```python
from build123d import *

# Parameters (mm, degrees)
SKETCH_1_W      = 180
SKETCH_1_H      = 98
SKETCH_1_R      = 6.2
SKETCH_1_R_2    = 8.2
SKETCH_1_R_3    = 1.5
SKETCH_1_R_4    = 1.75
SKETCH_1_R_5    = 3.6
SKETCH_1_R_6    = 3.8
SKETCH_1_W_2    = 12.5
SKETCH_1_H_2    = 12.5
SKETCH_1_W_3    = 46.5
SKETCH_1_H_3    = 36
EXTRUDE_1_DEPTH = 2.2
FILLET_1_R      = 1
FILLET_2_R      = 0.5


with BuildPart() as part:
    # Эскиз1 → Бобышка-Вытянуть1 (new body)
    with BuildSketch(Plane.XY):
        with Locations((49.911, 29.5)):
            Rectangle(SKETCH_1_W, SKETCH_1_H)
        with Locations((-24.089, 5.5)):
            Circle(SKETCH_1_R, mode=Mode.SUBTRACT)
        with Locations((123.911, 58.5)):
            Circle(SKETCH_1_R, mode=Mode.SUBTRACT)
        with Locations((123.911, 5.5)):
            Circle(SKETCH_1_R_2, mode=Mode.SUBTRACT)
        with Locations((-37.589, 76)):
            Circle(SKETCH_1_R_3, mode=Mode.SUBTRACT)
        with Locations((137.411, 76)):
            Circle(SKETCH_1_R_3, mode=Mode.SUBTRACT)
        with Locations((137.411, -17)):
            Circle(SKETCH_1_R_3, mode=Mode.SUBTRACT)
        with Locations((-37.589, -17)):
            Circle(SKETCH_1_R_3, mode=Mode.SUBTRACT)
        with Locations((3.556, 3.556)):
            Circle(SKETCH_1_R_4, mode=Mode.SUBTRACT)
        with Locations((3.556, 66.421)):
            Circle(SKETCH_1_R_4, mode=Mode.SUBTRACT)
        with Locations((96.266, 66.421)):
            Circle(SKETCH_1_R_4, mode=Mode.SUBTRACT)
        with Locations((96.266, 3.556)):
            Circle(SKETCH_1_R_4, mode=Mode.SUBTRACT)
        with Locations((8.255, 52.959)):
            Circle(SKETCH_1_R_5, mode=Mode.SUBTRACT)
        with Locations((91.567, 52.959)):
            Circle(SKETCH_1_R_5, mode=Mode.SUBTRACT)
        with Locations((-24.089, 30.5)):
            Circle(SKETCH_1_R_6, mode=Mode.SUBTRACT)
        with Locations((-24.089, -10.5)):
            Circle(SKETCH_1_R_6, mode=Mode.SUBTRACT)
        with Locations((38.7, 68)):
            Circle(SKETCH_1_R_3, mode=Mode.SUBTRACT)
        with Locations((16.891, 11.049)):
            Rectangle(SKETCH_1_W_2, SKETCH_1_H_2, mode=Mode.SUBTRACT)
        with Locations((38.1, 11.049)):
            Rectangle(SKETCH_1_W_2, SKETCH_1_H_2, mode=Mode.SUBTRACT)
        with Locations((61.722, 11.049)):
            Rectangle(SKETCH_1_W_2, SKETCH_1_H_2, mode=Mode.SUBTRACT)
        with Locations((82.931, 11.049)):
            Rectangle(SKETCH_1_W_2, SKETCH_1_H_2, mode=Mode.SUBTRACT)
        with Locations((49.75, 46)):
            Rectangle(SKETCH_1_W_3, SKETCH_1_H_3, mode=Mode.SUBTRACT)
        with BuildLine():
            Line((3.255, 36.5885), (13.255, 36.5885))
            ThreePointArc((13.255, 36.5885), (14.855, 34.9885), (13.255, 33.3885))
            Line((13.255, 33.3885), (3.255, 33.3885))
            ThreePointArc((3.255, 33.3885), (1.655, 34.9885), (3.255, 36.5885))
        make_face(mode=Mode.SUBTRACT)
        with BuildLine():
            Line((96.567, 33.3885), (86.567, 33.3885))
            ThreePointArc((86.567, 33.3885), (84.967, 34.9885), (86.567, 36.5885))
            Line((86.567, 36.5885), (96.567, 36.5885))
            ThreePointArc((96.567, 36.5885), (98.167, 34.9885), (96.567, 33.3885))
        make_face(mode=Mode.SUBTRACT)
        with BuildLine():
            Line((3.255, 32.5885), (13.255, 32.5885))
            ThreePointArc((13.255, 32.5885), (14.855, 30.9885), (13.255, 29.3885))
            Line((13.255, 29.3885), (3.255, 29.3885))
            ThreePointArc((3.255, 29.3885), (1.655, 30.9885), (3.255, 32.5885))
        make_face(mode=Mode.SUBTRACT)
        with BuildLine():
            Line((96.567, 29.3885), (86.567, 29.3885))
            ThreePointArc((86.567, 29.3885), (84.967, 30.9885), (86.567, 32.5885))
            Line((86.567, 32.5885), (96.567, 32.5885))
            ThreePointArc((96.567, 32.5885), (98.167, 30.9885), (96.567, 29.3885))
        make_face(mode=Mode.SUBTRACT)
        with BuildLine():
            Line((3.255, 28.5885), (13.255, 28.5885))
            ThreePointArc((13.255, 28.5885), (14.855, 26.9885), (13.255, 25.3885))
            Line((13.255, 25.3885), (3.255, 25.3885))
            ThreePointArc((3.255, 25.3885), (1.655, 26.9885), (3.255, 28.5885))
        make_face(mode=Mode.SUBTRACT)
        with BuildLine():
            Line((96.567, 25.3885), (86.567, 25.3885))
            ThreePointArc((86.567, 25.3885), (84.967, 26.9885), (86.567, 28.5885))
            Line((86.567, 28.5885), (96.567, 28.5885))
            ThreePointArc((96.567, 28.5885), (98.167, 26.9885), (96.567, 25.3885))
        make_face(mode=Mode.SUBTRACT)
        with BuildLine():
            Line((3.255, 24.5885), (13.255, 24.5885))
            ThreePointArc((13.255, 24.5885), (14.855, 22.9885), (13.255, 21.3885))
            Line((13.255, 21.3885), (3.255, 21.3885))
            ThreePointArc((3.255, 21.3885), (1.655, 22.9885), (3.255, 24.5885))
        make_face(mode=Mode.SUBTRACT)
        with BuildLine():
            Line((96.567, 21.3885), (86.567, 21.3885))
            ThreePointArc((86.567, 21.3885), (84.967, 22.9885), (86.567, 24.5885))
            Line((86.567, 24.5885), (96.567, 24.5885))
            ThreePointArc((96.567, 24.5885), (98.167, 22.9885), (96.567, 21.3885))
        make_face(mode=Mode.SUBTRACT)
    extrude(amount=EXTRUDE_1_DEPTH)

    # Скругление1
    fillet_1_edges = [part.edges().sort_by_distance(p)[0] for p in [
        (139.911, -19.5, 1.1),
        (-40.089, -19.5, 1.1),
        (-40.089, 78.5, 1.1),
        (139.911, 78.5, 1.1),
    ]]
    fillet(fillet_1_edges, radius=FILLET_1_R)

    # Скругление2
    fillet_2_edges = [part.edges().sort_by_distance(p)[0] for p in [
        (89.181, 4.799, 1.1),
        (89.181, 17.299, 1.1),
        (76.681, 17.299, 1.1),
        (76.681, 4.799, 1.1),
        (23.141, 4.799, 1.1),
        (23.141, 17.299, 1.1),
        (10.641, 17.299, 1.1),
        (10.641, 4.799, 1.1),
        (44.35, 4.799, 1.1),
        (44.35, 17.299, 1.1),
        (31.85, 17.299, 1.1),
        (31.85, 4.799, 1.1),
        (67.972, 4.799, 1.1),
        (67.972, 17.299, 1.1),
        (55.472, 17.299, 1.1),
        (55.472, 4.799, 1.1),
    ]]
    fillet(fillet_2_edges, radius=FILLET_2_R)


solid = part.part
```
Input: part model. Units: mm. Frame: model coordinates. Round coordinates to 2 decimals unless told otherwise and drop trailing zeros. Loops run counter-clockwise (first coordinate to the right, second up) from the corner with the lowest first, then second, coordinate; pieces in that order, holes last. Notation, with made-up numbers: (-28, -22.5) -> (26, -22.5) arc R11 ccw to (26, -16.5) -> close; hole circle Ø3 at (11.25, 40). An arc over 180 degrees is marked (long way). Use one line per item in the form item = value. Start each with the question number.
Item 1: Section query A-A on x = 59. Return the cut outline in (y, z), then the cut area to 3 significant figures.
Item 2: Mould query, pull axis X, two halves, no side actions, for faces 1 (the face through (94.518, 3.633, 1.085)), 2 (the face through (49, 19, 2.2)). Classes: pulls with the +X half, pulls with the -X half, needs draft (parallel to the pull), parting line crosses it, or undercut.
Item 3: Section query B-B on y = 43.5. Return the cut outline in (x, z), then the cut area to 3 significant figures.
Item 4: Section query D-D on y = -10.5. Return the cut outline in (x, z), then the cut area to 3 significant figures.
Item 5: Material intervals for L1, parallel to X at y = 59, z = 0.95; L2, parallel to Y at x = 41, z = 0.7; L3, parallel to X at y = 76, z = 0.5, sorted ascending. Write a range as from..to.
Item 6: Section query C-C on x = 92.5. Return the cut outline in (y, z).
Ans:
q1.outline = (-19.5, 0) -> (4.8, 0) -> (4.8, 2.2) -> (-19.5, 2.2) -> close; (17.3, 0) -> (28, 0) -> (28, 2.2) -> (17.3, 2.2) -> close; (64, 0) -> (78.5, 0) -> (78.5, 2.2) -> (64, 2.2) -> close
q1.area = 109 mm^2
q2.face_1 = undercut
q2.face_2 = needs draft
q3.outline = (-40.09, 0) -> (26.5, 0) -> (26.5, 2.2) -> (-40.09, 2.2) -> close; (73, 0) -> (139.91, 0) -> (139.91, 2.2) -> (73, 2.2) -> close
q3.area = 294 mm^2
q4.outline = (-40.09, 0) -> (-27.89, 0) -> (-27.89, 2.2) -> (-40.09, 2.2) -> close; (-20.29, 0) -> (139.91, 0) -> (139.91, 2.2) -> (-20.29, 2.2) -> close
q4.area = 379 mm^2
q5.L1 = -40.09..26.5, 73..117.73, 130.09..139.91
q5.L2 = -19.5..4.8, 17.3..28, 64..78.5
q5.L3 = -40.09..-39.09, -36.09..135.91, 138.91..139.91
q6.outline = (-19.5, 0) -> (21.39, 0) -> (21.39, 2.2) -> (-19.5, 2.2) -> close; (24.59, 0) -> (25.39, 0) -> (25.39, 2.2) -> (24.59, 2.2) -> close; (28.59, 0) -> (29.39, 0) -> (29.39, 2.2) -> (28.59, 2.2) -> close; (32.59, 0) -> (33.39, 0) -> (33.39, 2.2) -> (32.59, 2.2) -> close; (36.59, 0) -> (49.48, 0) -> (49.48, 2.2) -> (36.59, 2.2) -> close; (56.44, 0) -> (78.5, 0) -> (78.5, 2.2) -> (56.44, 2.2) -> close
